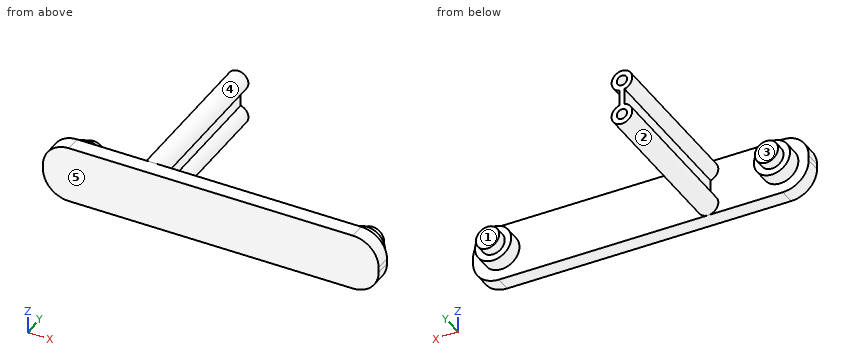
from build123d import *

# Parameters (mm, degrees)
SKETCH2_W           = 65
SKETCH2_H           = 11
BOSS_EXTRUDE1_DEPTH = 3
SKETCH2_4_R         = 3.5
SKETCH2_4_R_2       = 2.25
BOSS_EXTRUDE2_DEPTH = 3
SKETCH2_5_R         = 2.25
BOSS_EXTRUDE3_DEPTH = 5
SKETCH2_6_R         = 2
BOSS_EXTRUDE4_DEPTH = 31
FILLET1_R           = 5
SKETCH3_R           = 1
CUT_EXTRUDE1_DEPTH  = 10


with BuildPart() as part:
    # Sketch2 → Boss-Extrude1 (new body)
    with BuildSketch(Plane(origin=(0, 0, 0), x_dir=(1, 0, 0), z_dir=(0, 1, 0))):
        with Locations((-23.91453319, 13.570918432)):
            Rectangle(SKETCH2_W, SKETCH2_H)
    extrude(amount=-BOSS_EXTRUDE1_DEPTH)

    # Sketch2<4> → Boss-Extrude2 (add)
    with BuildSketch(Plane(origin=(0, 0, 0), x_dir=(1, 0, 0), z_dir=(0, 1, 0))):
        with Locations(Location((-50.91453319, 13.570918432, 0), (0, 0, 270))):
            Circle(SKETCH2_4_R)
        with Locations(Location((3.08546681, 13.570918432, 0), (0, 0, 270))):
            Circle(SKETCH2_4_R)
        with Locations((-50.91453319, 13.570918432)):
            Circle(SKETCH2_4_R_2)
        with Locations((3.08546681, 13.570918432)):
            Circle(SKETCH2_4_R_2)
    extrude(amount=BOSS_EXTRUDE2_DEPTH)

    # Sketch2<5> → Boss-Extrude3 (add)
    with BuildSketch(Plane(origin=(0, 0, 0), x_dir=(1, 0, 0), z_dir=(0, 1, 0))):
        with Locations(Location((-50.91453319, 13.570918432, 0), (0, 0, 270))):
            Circle(SKETCH2_5_R)
        with Locations(Location((3.08546681, 13.570918432, 0), (0, 0, 270))):
            Circle(SKETCH2_5_R)
    extrude(amount=BOSS_EXTRUDE3_DEPTH)

    # Sketch2<6> → Boss-Extrude4 (add)
    with BuildSketch(Plane(origin=(0, 0, 0), x_dir=(1, 0, 0), z_dir=(0, 1, 0))):
        with Locations((-36.91453319, 17.070918432)):
            Circle(SKETCH2_6_R)
        with Locations((-36.91453319, 10.070918432)):
            Circle(SKETCH2_6_R)
        with BuildLine():
            ThreePointArc((-36.41453319, 15.134426759), (-36.91453319, 15.070918432), (-37.41453319, 15.134426759))
            Line((-37.41453319, 15.134426759), (-37.41453319, 12.007410105))
            ThreePointArc((-37.41453319, 12.007410105), (-36.91453319, 12.070918432), (-36.41453319, 12.007410105))
            Line((-36.41453319, 12.007410105), (-36.41453319, 15.134426759))
        make_face()
    extrude(amount=BOSS_EXTRUDE4_DEPTH)

    # Fillet1
    fillet1_edges = [part.edges().sort_by_distance(p)[0] for p in [
        (-56.41453319, -1.5, -8.070918432),
        (-56.41453319, -1.5, -19.070918432),
        (8.58546681, -1.5, -19.070918432),
        (8.58546681, -1.5, -8.070918432),
    ]]
    fillet(fillet1_edges, radius=FILLET1_R)

    # Sketch3 → Cut-Extrude1 (cut)
    with BuildSketch(Plane(origin=(0, 31, 0), x_dir=(1, 0, 0), z_dir=(0, 1, 0))):
        with Locations(Location((-36.91453319, 10.070918432, 0), (0, 0, 270))):
            Circle(SKETCH3_R)
        with Locations(Location((-36.91453319, 17.070918432, 0), (0, 0, 270))):
            Circle(SKETCH3_R)
    extrude(amount=-CUT_EXTRUDE1_DEPTH, mode=Mode.SUBTRACT)


solid = part.part
The listing builds one solid part. Answer for the finished solid, in the listing's coordinates (mm). Face numbers are marked on the shaded views. A direction names the side the tool comes from. Round coordinates to 2 decimals unless told otherwise and drop trailing zeros. Write each loop counter-clockwise with the first axis right and the second up, starting at its lowest first coordinate (ties: lowest second). Pieces come first, ordered by that corner, then holes. Notation, with made-up numbers: (9, -27.5) - (42, -27.5) arc R22 ccw to (42, -10.5) - close; hole circle Ø11 at (53, 20). An arc over 180 degrees is marked (long way). Use one line per item in the form item = value. Start each with the question number.
Item 1: Find the intervals of material crossed by line 1 (Z direction, x = -37, y = 22); line 2 (X direction, y = 4, z = -15); line 3 (Y direction, x = -41, z = -16.5), in increasing order. Write a range as [from, to].
Item 2: Determine the mould class of the marked faces 4 and 5 for opening direction Z: +Z half, -Z half, draft (parallel to the pull), parting line (faces both ways), or undercut.
Item 3: A cutting plane is placed at C-C (y = 13.5). Write down the section's boundary in (x, z).
Item 4: A tool of negligible diameter and unlimited length cuts with its end or side. For the marked faces 1, 2 and 3, from which of +Z, -Z, +X, -X, +Y, -Y can it reach the whole face along a straight path? Write none if from no direction.
Item 5: A cutting plane is placed at A-A (y = 24). Write down the section's boundary in (x, z), plus the area to 3 significant figures.
Item 6: A cutting plane is placed at D-D (x = -13.5). Write down the section's boundary in (y, z), plus the area to 3 significant figures.
Item 7: A cutting plane is placed at B-B (x = 4.5). Write down the section's boundary in (y, z).
Item 8: Flat-ended cylindrical pins translate along their axes: pin 1 Ø2 at (x, z) = (-37, -17.5) entering from +Y; pin 2 Ø1.5 at (y, z) = (10.5, -15) entering from -X; pin 3 Ø1.5 at (y, z) = (6.5, -17) entering from +X; pin 4 Ø3 at (y, z) = (19, -14.5) entering from +X. Find the tip coordinate at first contact, or state that the pin passes through.
The answers:
q1.line_1 = [-19.07, -18.07], [-16.07, -11.07], [-9.07, -8.07]
q1.line_2 = [-52.65, -49.18], [-37.41, -36.41], [1.35, 4.82]
q1.line_3 = [-3, 0]
q2.face_4 = undercut
q2.face_5 = draft
q3.outline = (-37.41, -15.13) arc R2 ccw (long way) to (-36.41, -15.13) - (-36.41, -12.01) arc R2 ccw (long way) to (-37.41, -12.01) - close
q4.face_1 = +Z, -Z, +X, +Y
q4.face_2 = +Y
q4.face_3 = +Z, -Z, -X, +Y
q5.outline = (-37.41, -15.13) arc R2 ccw (long way) to (-36.41, -15.13) - (-36.41, -12.01) arc R2 ccw (long way) to (-37.41, -12.01) - close; hole circle Ø2 at (-36.91, -17.07); hole circle Ø2 at (-36.91, -10.07)
q5.area = 21.9 mm^2
q6.outline = (-3, -19.07) - (0, -19.07) - (0, -8.07) - (-3, -8.07) - close
q6.area = 33.0 mm^2
q7.outline = (-3, -18.99) - (0, -18.99) - (0, -16.77) - (3, -16.77) - (3, -15.32) - (5, -15.32) - (5, -11.82) - (3, -11.82) - (3, -10.37) - (0, -10.37) - (0, -8.16) - (-3, -8.16) - close
q8.pin_1 = 31
q8.pin_2 = -38.42
q8.pin_3 = -34.91
q8.pin_4 = -35.23
